Answer from the drawing. Dimensions are ordinates in mm from the lowest x, y and z of the part. A direction names the side the tool comes from. Round coordinates to 2 decimals unless told otherwise and drop trailing zeros. Write each loop counter-clockwise with the first axis right and the second up, starting at its lowest first coordinate (ties: lowest second). Pieces come first, ordered by that corner, then holes. Notation, with made-up numbers: (29, 42.5) - (53, 42.5) arc R23 cw to (53, 65.5) - close; hole circle Ø7 at (60.25, 2). An arc over 180 degrees is marked (long way). Use a Markdown table: item, result. Add a question column.
1) Determine the mould class of the marked faces 3, 4 and 5 for opening direction X: +X half, -X half, draft (parallel to the pull), parting line (faces both ways), or undercut.
2) Each of these flat-tipped pins is pushed along its axis until it touches: P1, Ø5, axis at x = 96, y = 33, coming from the +Z side; P2, Ø4, axis at x = 80, y = 56, coming from the +Z side; P3, Ø3, axis at x = 82.5, z = 57, coming from the -Y side; P4, Ø3, axis at x = 89, z = 39, coming from the +Y side (1 decimal). Where does it stop, or does it pass through?
3) A cutting plane is placed at D-D (x = 93). Give the vertices of the cut face in (y, z).
4) A cutting plane is placed at B-B (z = 31). Give the vertices of the cut face in (x, y) (1 decimal), then the cut area to 3 significant figures.
5) A tool of negligible diameter and unlimited length cuts with its end or side. For the marked faces 1 and 2, from which of +Z, -Z, +X, -X, +Y, -Y can it reach the whole face along a straight path? Write none if from no direction.
6) A cutting plane is placed at A-A (y = 62). Give the vertices of the cut face in (x, z), then the cut area to 4 significant figures.
7) A cutting plane is placed at C-C (z = 48.5). Give the vertices of the cut face in (x, y).
8) Find the intervals of material crossed by probe 1 along X at (y, z) = (98, 25.5); probe 2 along X at (y, z) = (110.5, 26); probe 3 along X at (y, z) = (66.5, 53), in increasing order. Write a range as from..to.
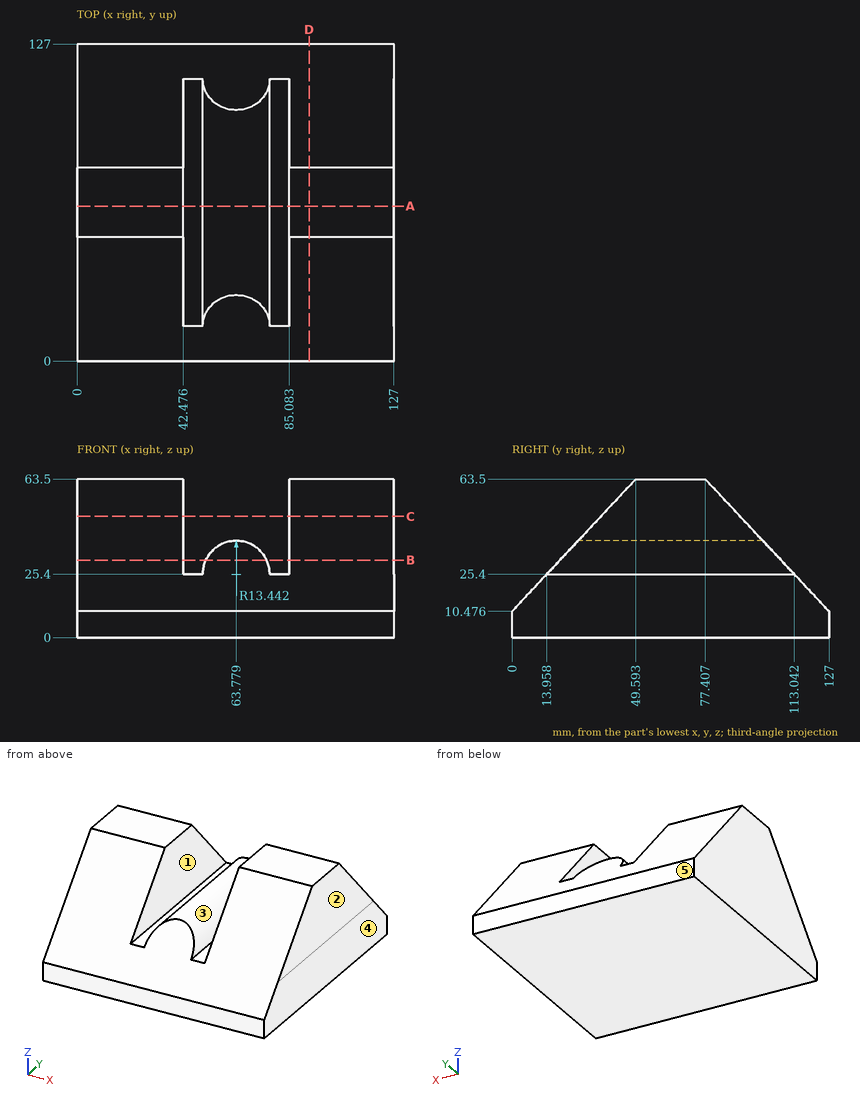
Entries:
| question | item | result |
|---|---|---|
| 1 | face 3 | undercut |
| 1 | face 4 | +X half |
| 1 | face 5 | draft |
| 2 | P1 | stops at z = 48.43 |
| 2 | P2 | stops at z = 25.4 |
| 2 | P3 | passes through |
| 2 | P4 | stops at y = 101.7 |
| 3 | outline | (0, 0) - (127, 0) - (127, 10.48) - (77.41, 63.5) - (49.59, 63.5) - (0, 10.48) - close |
| 4 | outline | (0, 19.2) - (42.5, 19.2) - (42.5, 107.8) - (0, 107.8) - close; (51.6, 19.2) - (76, 19.2) - (76, 107.8) - (51.6, 107.8) - close; (85.1, 19.2) - (127, 19.2) - (127, 107.8) - (85.1, 107.8) - close |
| 4 | area | 9,640 mm² |
| 5 | face 1 | +Z, +Y, -Y |
| 5 | face 2 | +Z, -Z, +X, +Y, -Y |
| 6 | outline | (0, 0) - (127, 0) - (127, 63.5) - (85.08, 63.5) - (85.08, 25.4) - (77.22, 25.4) arc R13.44 ccw to (50.34, 25.4) - (42.48, 25.4) - (42.48, 63.5) - (0, 63.5) - close |
| 6 | area | 6,725 mm² |
| 7 | outline | (0, 35.56) - (42.48, 35.56) - (42.48, 91.44) - (0, 91.44) - close; (85.08, 35.56) - (127, 35.56) - (127, 91.44) - (85.08, 91.44) - close |
| 8 | probe 1 | x = 0..42.48, 50.34..77.22, 85.08..127 |
| 8 | probe 2 | x = 0..42.48, 50.35..77.21, 85.08..127 |
| 8 | probe 3 | x = 0..42.48, 85.08..127 |
